For this review, take the finished solid that the model builds, in its own axes (mm). Round coordinates to 2 decimals unless told otherwise and drop trailing zeros. Write each loop counter-clockwise with the first axis right and the second up, starting at its lowest first coordinate (ties: lowest second). Pieces come first, ordered by that corner, then holes. Notation, with made-up numbers: (-9.75, 56) -> (8.25, 56) arc R26 cw to (8.25, 93) -> close; hole circle Ø5 at (36.25, 40.5). An arc over 180 degrees is marked (long way). Answer in a Markdown table with one row per item.
from build123d import *

# Parameters (mm, degrees)
F1_DEPTH = 25.4
F3_D     = 12.7
F3_DEPTH = 254
F3_TIP   = 3.8154649308
F4_W     = 25.4
F4_H     = 82.55
F5_DEPTH = 25.4
F7_DEPTH = 25.4
F8_R     = 6.34999


# Not quite as in the source:
# - a fillet or chamfer is up to 0.001 mm smaller than in the source, because OpenCascade refuses the exact size


with BuildPart() as f1:
    # F0 (on Front) → F1 (new body)
    with BuildSketch(Plane.XZ):
        Polygon((-12.7, -32.0098340811), (0, -32.0098340811), (12.7, -32.0098340811), (12.7, 69.5901659189), (-12.7, 69.5901659189), align=None)
    extrude(amount=F1_DEPTH)

    # F3
    with Locations(Plane.XZ.offset(25.4)):
        with Locations((0, 56.8901659189), (0, -19.3098340811)):
            Hole(F3_D / 2, depth=F3_DEPTH)
            with Locations((0, 0, -(F3_DEPTH + F3_TIP / 2))):  # 118° drill point
                Cone(0, F3_D / 2, F3_TIP, mode=Mode.SUBTRACT)

    # F4 (on face) → F5 (join)
    with BuildSketch(Plane.XZ.offset(25.4)):
        with Locations((0, -73.2848340811)):
            Rectangle(F4_W, F4_H)
    extrude(amount=-F5_DEPTH)

    # F6 (on face) → F7 (cut)
    with BuildSketch(Plane(origin=(0, 0, 0), x_dir=(-1, 0, 0), z_dir=(0, 1, 0))):
        Polygon((0, -105.6698340811), (6.35, -105.6698340811), (6.35, -92.9698340811), (-6.35, -92.9698340811), (-6.35, -105.6698340811), align=None)
    extrude(amount=-F7_DEPTH, mode=Mode.SUBTRACT)

    # F8 (radius 6.35 in the source; OpenCascade refuses exactly that, so slightly less here)
    f8_edges = [f1.edges().sort_by_distance(p)[0] for p in [
        (12.7, 0, -22.484834),
        (-12.7, 0, -22.484834),
        (-12.7, -25.4, -22.484834),
        (12.7, -25.4, -22.484834),
    ]]
    fillet(f8_edges, radius=F8_R)


solid = f1.part
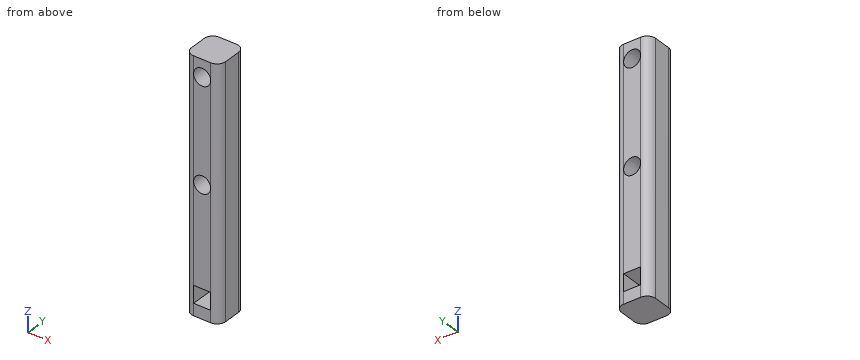
1) Clearance check with flat-ended pins moving along their axes: pin 1 Ø10 at (x, z) = (0, 56.89) entering from -Y; pin 2 Ø3 at (x, z) = (8, 16.5) entering from +Y. State where each tip first meets the part, or that it passes through.
Solved:
| item | result |
|---|---|
| pin 1 | through |
| pin 2 | y = 0 |
2) For line 1 (Z direction, x = 0, y = -16); line 2 (Z direction, x = -5, y = -8.5); line 3 (X direction, y = -22.25, z = -99.5), list the stretches that pass through material, from the lowest coordinate up. Write a range as [from, to].
Solved:
| item | result |
|---|---|
| line 1 | [-114.56, -105.67], [-92.97, -25.66], [-12.96, 50.54], [63.24, 69.59] |
| line 2 | [-114.56, -105.67], [-92.97, -23.22], [-15.4, 52.98], [60.8, 69.59] |
| line 3 | [-11.83, -6.35], [6.35, 11.83] |
3) Consider section B-B on z = -66.5. State the section outline as (x, y) points, then the cut area to 3 significant figures.
Solved:
| item | result |
|---|---|
| outline | (-12.7, -19.05) arc R6.35 ccw to (-6.35, -25.4) -> (6.35, -25.4) arc R6.35 ccw to (12.7, -19.05) -> (12.7, -6.35) arc R6.35 ccw to (6.35, 0) -> (-6.35, 0) arc R6.35 ccw to (-12.7, -6.35) -> close |
| area | 611 mm² |
4) Consider section C-C on x = 8.75. State the section outline as (y, z) points, then the cut area to 3 significant figures.
Solved:
| item | result |
|---|---|
| outline | (-24.93, -114.56) -> (-0.47, -114.56) -> (-0.47, 69.59) -> (-24.93, 69.59) -> close |
| area | 4,500 mm² |
5) Consider section A-A on x = 0. State the section outline as (y, z) points, then the cut area to 3 significant figures.
Solved:
| item | result |
|---|---|
| outline | (-25.4, -114.56) -> (0, -114.56) -> (0, -105.67) -> (-25.4, -105.67) -> close; (-25.4, -92.97) -> (0, -92.97) -> (0, -25.66) -> (-25.4, -25.66) -> close; (-25.4, -12.96) -> (0, -12.96) -> (0, 50.54) -> (-25.4, 50.54) -> close; (-25.4, 63.24) -> (0, 63.24) -> (0, 69.59) -> (-25.4, 69.59) -> close |
| area | 3,710 mm² |
